Read the model definition and answer for the solid it produces. Units are mm, in the model's axes. Give positions to 0.01 mm unless a question says otherwise; leave off trailing zeros. Loops run counter-clockwise (first coordinate to the right, second up) from the corner with the lowest first, then second, coordinate; pieces in that order, holes last. Notation, with made-up numbers: (40.25, 58.25) -> (66.25, 58.25) arc R23 cw to (66.25, 86.25) -> close; hole circle Ø11 at (-40, 30). An arc over 180 degrees is marked (long way). Write each question's results on one line, items separated by ' | '. Start each with the question number.
Item 1: Find the intervals of material crossed by line 1 (X direction, y = 67.5, z = 0.7); line 2 (Y direction, x = 315, z = 0.8); line 3 (X direction, y = 59, z = 0.7), in increasing order.
Item 2: Section C-C on y = 52 is taken. Write down the section's boundary in (x, z).
Item 3: Each of these flat-tipped pins is pushed along its axis until it touches: P1, Ø1.5, axis at x = 316, z = 0.5, coming from the -Y side; P2, Ø1, axis at x = 289.5, z = 2, coming from the -Y side; P3, Ø1.5, axis at y = 37.5, z = 2, coming from the +X side. Where does it stop, or does it pass through?
Item 4: Section B-B on x = 317 is taken. Write down the section's boundary in (y, z), and give its area (3 significant figures).
Item 5: Section D-D on x = 299 is taken. Write down the section's boundary in (y, z), and give its area (3 significant figures).
Item 6: Section A-A on z = 2.15 is taken. Write down the section's boundary in (x, y).
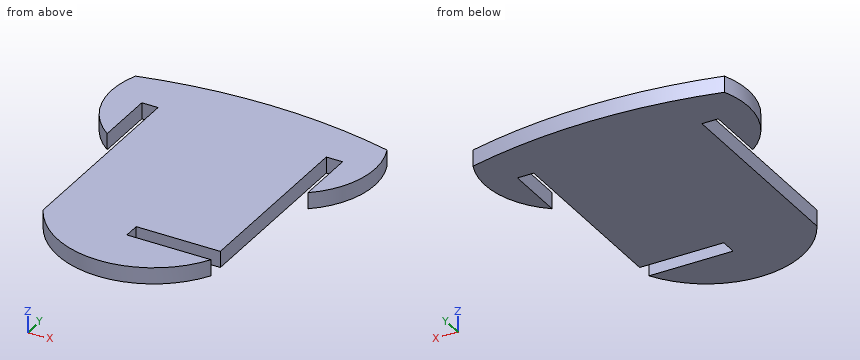
```python
from build123d import *

# Parameters (mm, degrees)
BASE_EXTRUDE_DEPTH = 3


with BuildPart() as part:
    # Sketch1 → Base-Extrude (new body)
    with BuildSketch(Plane.XY):
        with BuildLine():
            Line((327.434465654, 72.761168779), (327.434465654, 61.638791555))
            ThreePointArc((327.434465654, 61.638791555), (332.635220006, 69.823914354), (331.761917416, 79.482145231))
            ThreePointArc((331.761917416, 79.482145231), (308.592008451, 82.313990162), (285.421828233, 79.484365486))
            ThreePointArc((285.421828233, 79.484365486), (284.853925586, 69.698061489), (290.434465654, 61.638791555))
            Line((290.434465654, 61.638791555), (290.434465654, 72.761168779))
            Line((290.434465654, 72.761168779), (293.434465654, 72.761168779))
            Line((293.434465654, 72.761168779), (293.434465654, 35.847162793))
            ThreePointArc((293.434465654, 35.847162793), (308.912610373, 26.65368117), (324.434465654, 35.773170023))
            Line((324.434465654, 35.773170023), (308.934465654, 35.773170023))
            Line((308.934465654, 35.773170023), (308.934465654, 38.773170023))
            Line((308.934465654, 38.773170023), (324.434465654, 38.773170023))
            Line((324.434465654, 38.773170023), (324.434465654, 72.761168779))
            Line((324.434465654, 72.761168779), (327.434465654, 72.761168779))
        make_face()
    extrude(amount=BASE_EXTRUDE_DEPTH)


solid = part.part
```
Findings:
1) line 1: 285.66 to 290.43, 293.43 to 324.43, 327.43 to 331.87 | line 2: 27.72 to 35.77, 38.77 to 82.1 | line 3: 293.43 to 324.43
2) outline: (293.43, 0) -> (324.43, 0) -> (324.43, 3) -> (293.43, 3) -> close
3) P1: y = 27.81 | P2: y = 61.97 | P3: x = 308.93
4) outline: (28.59, 0) -> (35.77, 0) -> (35.77, 3) -> (28.59, 3) -> close; (38.77, 0) -> (81.95, 0) -> (81.95, 3) -> (38.77, 3) -> close | area: 151 mm2
5) outline: (29.72, 0) -> (81.84, 0) -> (81.84, 3) -> (29.72, 3) -> close | area: 156 mm2
6) outline: (285.42, 79.48) arc R15.05 ccw to (290.43, 61.64) -> (290.43, 72.76) -> (293.43, 72.76) -> (293.43, 35.85) arc R17.7 ccw to (324.43, 35.77) -> (308.93, 35.77) -> (308.93, 38.77) -> (324.43, 38.77) -> (324.43, 72.76) -> (327.43, 72.76) -> (327.43, 61.64) arc R15.05 ccw to (331.76, 79.48) arc R96.24 ccw to start
